Geometry: final body of the model. Coordinates: model frame, mm. A direction names the side the tool comes from. Give positions to 0.01 mm unless a question says otherwise; leave off trailing zeros. Write each loop counter-clockwise with the first axis right and the second up, starting at its lowest first coordinate (ties: lowest second). Pieces come first, ordered by that corner, then holes. Notation, with made-up numbers: (-39.5, 49) -> (-18.5, 49) arc R11 cw to (-18.5, 60) -> close; hole circle Ø11 at (-20.5, 33). An arc over 180 degrees is marked (long way). Answer as a JSON object with one key per item and string values.
from build123d import *

# Parameters (mm, degrees)
SKETCH1_W               = 29.275000124
SKETCH1_H               = 44.45
BOSS_EXTRUDE1_DEPTH     = 3
SKETCH2_W               = 3
SKETCH2_H               = 6.35
BOSS_EXTRUDE2_DEPTH     = 6
LPATTERN1_COUNT         = 3
LPATTERN1_PITCH         = 12.7
MIRROR1_COPY_1_SKETCH_W = 3
MIRROR1_COPY_1_SKETCH_H = 6.35
MIRROR1_COPY_1_DEPTH    = 6
MIRROR1_COPY_2_SKETCH_W = 3
MIRROR1_COPY_2_SKETCH_H = 6.35
MIRROR1_COPY_2_DEPTH    = 6
FILLET1_R               = 1.27


with BuildPart() as part:
    # Sketch1 → Boss-Extrude1 (new body)
    with BuildSketch(Plane.XY):
        Rectangle(SKETCH1_W, SKETCH1_H)
    extrude(amount=BOSS_EXTRUDE1_DEPTH)

    # Sketch2 → Boss-Extrude2 (add)
    with BuildSketch(Plane(origin=(14.637500062, 0, 0), x_dir=(0, 0, -1), z_dir=(1, 0, 0))):
        with Locations((-1.5, -12.7)):
            Rectangle(SKETCH2_W, SKETCH2_H)
    boss_extrude2 = extrude(amount=BOSS_EXTRUDE2_DEPTH)

    # LPattern1: Boss-Extrude2 ×3
    with Locations(*[(0, i * LPATTERN1_PITCH, 0) for i in range(1, LPATTERN1_COUNT)]):
        add(boss_extrude2)

    # Mirror1: Boss-Extrude2 across plane
    add(boss_extrude2.mirror(Plane(origin=(0, 0, 0), x_dir=(0, 0, 1), z_dir=(1, 0, 0))))

    # Mirror1 copy 1 sketch → Mirror1 copy 1 (add)
    with BuildSketch(Plane(origin=(-14.637500062, 12.7, 0), x_dir=(0, 0, -1), z_dir=(-1, 0, 0))):
        with Locations((-1.5, 12.7)):
            Rectangle(MIRROR1_COPY_1_SKETCH_W, MIRROR1_COPY_1_SKETCH_H)
    extrude(amount=MIRROR1_COPY_1_DEPTH)

    # Mirror1 copy 2 sketch → Mirror1 copy 2 (add)
    with BuildSketch(Plane(origin=(-14.637500062, 25.4, 0), x_dir=(0, 0, -1), z_dir=(-1, 0, 0))):
        with Locations((-1.5, 12.7)):
            Rectangle(MIRROR1_COPY_2_SKETCH_W, MIRROR1_COPY_2_SKETCH_H)
    extrude(amount=MIRROR1_COPY_2_DEPTH)

    # Fillet1
    fillet1_edges = [part.edges().sort_by_distance(p)[0] for p in [
        (20.637500062, -15.875, 1.5),
        (20.637500062, -9.525, 1.5),
        (20.637500062, -3.175, 1.5),
        (20.637500062, 3.175, 1.5),
        (20.637500062, 9.525, 1.5),
        (20.637500062, 15.875, 1.5),
        (-20.637500062, -9.525, 1.5),
        (-20.637500062, -15.875, 1.5),
        (-20.637500062, 3.175, 1.5),
        (-20.637500062, -3.175, 1.5),
        (-20.637500062, 15.875, 1.5),
        (-20.637500062, 9.525, 1.5),
    ]]
    fillet(fillet1_edges, radius=FILLET1_R)


solid = part.part
Q1. Mould query, pull axis Y, two halves, no side actions, for faces 1 (the flat face through (17, -15.875, 2)), 2 (the cylindrical face through (-20.28, -2.79, 1.48)), 3 (the flat face through (0, 22.225, 1)), 4 (the flat face through (0, 0, 0)). Classes: pulls with the +Y half, pulls with the -Y half, needs draft (parallel to the pull), parting line crosses it, or undercut.
Values:
{"face 1": "pulls with the -Y half", "face 2": "undercut", "face 3": "pulls with the +Y half", "face 4": "needs draft"}
Q2. First-contact query: P1, Ø1.5, axis at y = -7, z = 1.5, coming from the -X side; P2, Ø1.5, axis at x = 17.5, z = 1.5, coming from the -Y side (3 decimals); P3, Ø1.5, axis at x = 17, z = 1, coming from the +Y side (3 decimals). Flat tips, straight axial feed; report the tip coordinate or a pass-through.
Values:
{"P1": "x = -14.64", "P2": "y = -15.875", "P3": "y = 15.875"}
Q3. Set-up query: faces 5 (the flat face through (-14.638, 19, 1)), 6 (the cylindrical face through (20.26, -2.81, 1.48)), 7 (the flat face through (-14.638, -19, 1)). Return all of +Z, -Z, +X, -X, +Y, -Y with unobstructed straight access to the full face (end or side cutting, diameter ignored); none if empty.
Values:
{"face 5": "+Z, -Z, -X, +Y", "face 6": "+Z, -Z, +X", "face 7": "+Z, -Z, -X, -Y"}
Q4. Cut plane A-A (y = -6). Return the cut outline in (x, z), and give its area (3 significant figures).
Values:
{"outline": "(-14.64, 0) -> (14.64, 0) -> (14.64, 3) -> (-14.64, 3) -> close", "area": "87.8 mm²"}
Q5. Material intervals for L1, parallel to Y at x = 18.5, z = 1.75 (3 decimals); L2, parallel to X at y = 9, z = 2.8; L3, parallel to X at y = -3, z = 1.3, sorted ascending. Write a range as from..to.
Values:
{"L1": "-15.875..-9.525, -3.175..3.175, 9.525..15.875", "L2": "-14.64..14.64", "L3": "-20.01..20.01"}
